Check sheet for the drawn part. Datum: minimum x, y, z corner. Units: mm. Round coordinates to 2 decimals unless told otherwise and drop trailing zeros. Write each loop counter-clockwise with the first axis right and the second up, starting at its lowest first coordinate (ties: lowest second). Pieces come first, ordered by that corner, then holes. Notation, with made-up numbers: M 62,10 L 68,10 A31 cw 68,47 Z; hole C 12.5,72 d8. An arc over 180 degrees is marked long. Use a Markdown table: item, result.
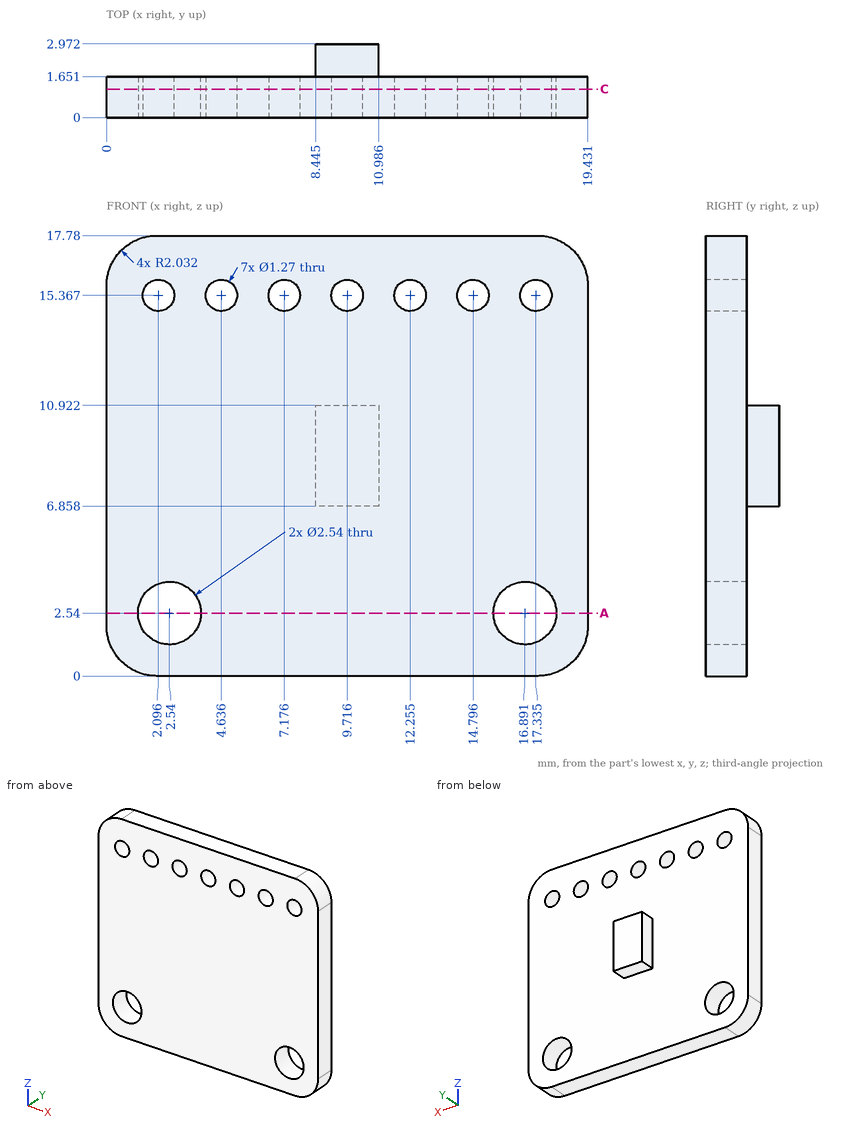
Item 1: Material ranges on line 1 along X through (y, z) = (1.1, 2.5); line 2 along Y through (x, z) = (1.25, 4); line 3 along X through (y, z) = (2, 10) (1 decimal), recorded low to high. Write a range as from..to.
Outcome:
| item | result |
|---|---|
| line 1 | x = 0..1.27, 3.81..15.62, 18.16..19.43 |
| line 2 | y = 0..1.65 |
| line 3 | x = 8.4..11 |
Item 2: Go/stop test with flat-tipped pins: pin 1 (1.1 mm diameter, centred on x = 10, y = 2.5, fed in from +Z); pin 2 (1.1 mm diameter, centred on x = 14.8, z = 15.37, fed in from -Y); pin 3 (2 mm diameter, centred on x = 4.64, z = 15.37, fed in from +Y). Record where each tip stops, or that it passes through.
Outcome:
| item | result |
|---|---|
| pin 1 | stops at z = 10.92 |
| pin 2 | passes through |
| pin 3 | stops at y = 1.65 |
Item 3: Cross-section at C-C, the plane y = 1.15. Count the separate pieces of the cut face and the enclosed holes in it, and give its area (3 significant figures).
Outcome:
| item | result |
|---|---|
| separate pieces | 1 |
| enclosed holes | 9 |
| area | 323 mm2 |
Item 4: Cross-section at A-A, the plane z = 2.54. Record the cut outline in (x, y), and give its area (3 significant figures).
Outcome:
| item | result |
|---|---|
| outline | M 0,0 L 1.27,0 L 1.27,1.65 L 0,1.65 Z; M 3.81,0 L 15.62,0 L 15.62,1.65 L 3.81,1.65 Z; M 18.16,0 L 19.43,0 L 19.43,1.65 L 18.16,1.65 Z |
| area | 23.7 mm2 |
